from build123d import *
from OCP.BRepFilletAPI import BRepFilletAPI_MakeChamfer

# Parameters (mm, degrees)
ESBO_O1_W                = 16.6
ESBO_O1_H                = 16.6
RESSALTO_EXTRUS_O1_DEPTH = 40
ESBO_O2_W                = 50
ESBO_O2_H                = 65
RESSALTO_EXTRUS_O2_DEPTH = 50
ESBO_O3_W                = 30
ESBO_O3_H                = 40
CORTE_EXTRUS_O1_DEPTH    = 86.732140997
ESBO_O4_R                = 11.5
ESBO_O4_R_2              = 2.5
CORTE_EXTRUS_O2_DEPTH    = 78.821912081
ESBO_O5_W                = 18
ESBO_O5_H                = 5
CORTE_EXTRUS_O3_DEPTH    = 10
CHANFRO1_SIZE            = 25
CHANFRO1_SIZE2           = 16.23518983
FILETE2_R                = 10
ESBO_O8_W                = 18
ESBO_O8_H                = 5
CORTE_EXTRUS_O5_DEPTH    = 30
FILETE4_R                = 10
ESBO_O9_R                = 2.5
CORTE_EXTRUS_O7_DEPTH    = 70.207225056


with BuildPart() as part:
    # Esboço1 → Ressalto-extrusão1 (new body)
    with BuildSketch(Plane(origin=(0, 0, 0), x_dir=(1, 0, 0), z_dir=(0, 1, 0))):
        Rectangle(ESBO_O1_W, ESBO_O1_H)
    extrude(amount=RESSALTO_EXTRUS_O1_DEPTH)

    # Esboço2 → Ressalto-extrusão2 (add)
    with BuildSketch(Plane.XZ):
        Rectangle(ESBO_O2_W, ESBO_O2_H)
    extrude(amount=RESSALTO_EXTRUS_O2_DEPTH)

    # Esboço3 → Corte-extrusão1 (cut, through all)
    with BuildSketch(Plane.XY.offset(32.5)):
        with Locations((0, -30)):
            Rectangle(ESBO_O3_W, ESBO_O3_H)
    extrude(amount=-CORTE_EXTRUS_O1_DEPTH, mode=Mode.SUBTRACT)

    # Esboço4 → Corte-extrusão2 (cut, through all)
    with BuildSketch(Plane(origin=(25, 0, 0), x_dir=(0, 0, -1), z_dir=(1, 0, 0))):
        with Locations((0, -22)):
            Circle(ESBO_O4_R)
        with Locations((-23.8125, -22)):
            Circle(ESBO_O4_R_2)
        with Locations((23.8125, -22)):
            Circle(ESBO_O4_R_2)
        with Locations((-11.90625, -42.622229928)):
            Circle(ESBO_O4_R_2)
        with Locations((11.90625, -42.622229928)):
            Circle(ESBO_O4_R_2)
    extrude(amount=-CORTE_EXTRUS_O2_DEPTH, mode=Mode.SUBTRACT)

    # Esboço5 → Corte-extrusão3 (cut)
    with BuildSketch(Plane.ZY.offset(25)):
        with Locations((-23.5, -2.5)):
            Rectangle(ESBO_O5_W, ESBO_O5_H)
    extrude(amount=-CORTE_EXTRUS_O3_DEPTH, mode=Mode.SUBTRACT)

    # Chanfro1: one chamfer whose edges measure the first distance from different faces: ONE call of the kernel's chamfer builder (chamfer() names one face for all edges)
    chanfro1_edges_1 = [part.edges().sort_by_distance(p)[0] for p in [
        (20, -50, 32.5),
        (-20, -50, 32.5),
    ]]
    chanfro1_side_1 = [part.faces().sort_by_distance(p)[0] for p in [
        (0, -0.707106781, 32.5),
    ]]
    chanfro1_edges_2 = [part.edges().sort_by_distance(p)[0] for p in [
        (-20, -50, -32.5),
        (20, -50, -32.5),
    ]]
    chanfro1_side_2 = [part.faces().sort_by_distance(p)[0] for p in [
        (5, -0.707106781, -32.5),
    ]]
    chanfro1 = BRepFilletAPI_MakeChamfer(part.part.solid().wrapped)
    for e in chanfro1_edges_1:
        chanfro1.Add(CHANFRO1_SIZE, CHANFRO1_SIZE2, e.wrapped, chanfro1_side_1[0].wrapped)  # the first distance lies on this face
    for e in chanfro1_edges_2:
        chanfro1.Add(CHANFRO1_SIZE, CHANFRO1_SIZE2, e.wrapped, chanfro1_side_2[0].wrapped)  # the first distance lies on this face
    add(Compound.cast(chanfro1.Shape()), mode=Mode.REPLACE)

    # Filete2
    # the kernel refuses this fillet: 10 mm, written as the material it takes off along each edge
    with BuildSketch(Plane(origin=(7.594662626, -25, -32.5), x_dir=(0, 1, 0), z_dir=(1, 0, 0)), Plane(origin=(-32.405337374, -25, -32.5), x_dir=(0, 1, 0), z_dir=(1, 0, 0)), Plane(origin=(32.405337374, -25, 32.5), x_dir=(0, 1, 0), z_dir=(-1, 0, 0)), Plane(origin=(-7.594662626, -25, 32.5), x_dir=(0, 1, 0), z_dir=(-1, 0, 0))) as filete2_piece_1:
        with BuildLine():
            CenterArc((FILETE2_R * 0.296213494962, FILETE2_R), FILETE2_R, 237, 33)
            Line((-FILETE2_R * 0.248425540053, FILETE2_R * 0.161329432055), (0, 0))
            Line((0, 0), (FILETE2_R * 0.296213494962, 0))
        make_face()
    extrude(amount=24.810674748, mode=Mode.SUBTRACT)
    with BuildSketch(Plane(origin=(1.426107509, -50, -16.26481017), x_dir=(0, 0.8386705679454236, -0.5446390350150278), z_dir=(1, 0, 0)), Plane(origin=(-1.426107509, -50, 16.26481017), x_dir=(0, 0.8386705679454233, 0.5446390350150284), z_dir=(-1, 0, 0)), Plane(origin=(-38.573892491, -50, -16.26481017), x_dir=(0, 0.8386705679454236, -0.5446390350150278), z_dir=(1, 0, 0))) as filete2_piece_2:
        with BuildLine():
            CenterArc((FILETE2_R * 0.542955699638, FILETE2_R), FILETE2_R, 213, 57)
            Line((-FILETE2_R * 0.295714868307, FILETE2_R * 0.455360964985), (0, 0))
            Line((0, 0), (FILETE2_R * 0.542955699638, 0))
        make_face()
    extrude(amount=37.147784982, mode=Mode.SUBTRACT)
    with BuildSketch(Plane(origin=(38.573892491, -50, 16.26481017), x_dir=(0, 0, -1), z_dir=(-1, 0, 0))) as filete2_piece_3:
        with BuildLine():
            CenterArc((FILETE2_R * 0.542955699638, -FILETE2_R), FILETE2_R, 90, 57)
            Line((-FILETE2_R * 0.295714868307, -FILETE2_R * 0.455360964985), (0, 0))
            Line((0, 0), (FILETE2_R * 0.542955699638, 0))
        make_face()
    extrude(amount=37.147784982, mode=Mode.SUBTRACT)
    with BuildSketch(Plane(origin=(50, 0, 32.5), x_dir=(0, 0, -1), z_dir=(-1, 0, 0))) as filete2_piece_4:
        with BuildLine():
            CenterArc((FILETE2_R, FILETE2_R), FILETE2_R, 180, 90)
            Line((0, FILETE2_R), (0, 0))
            Line((0, 0), (FILETE2_R, 0))
        make_face()
    extrude(amount=100, mode=Mode.SUBTRACT)
    with BuildSketch(Plane(origin=(-50, -5, -32.5), x_dir=(0, -1, 0), z_dir=(1, 0, 0))) as filete2_piece_5:
        with BuildLine():
            CenterArc((FILETE2_R, -FILETE2_R), FILETE2_R, 90, 90)
            Line((0, -FILETE2_R), (0, 0))
            Line((0, 0), (FILETE2_R, 0))
        make_face()
    extrude(amount=35, mode=Mode.SUBTRACT)

    # Esboço8 → Corte-extrusão5 (cut)
    with BuildSketch(Plane.ZY.offset(15)):
        with Locations((-23.5, -2.5)):
            Rectangle(ESBO_O8_W, ESBO_O8_H)
        with Locations((-23.5, -7.5)):
            Rectangle(ESBO_O8_W, ESBO_O8_H)
    extrude(amount=-CORTE_EXTRUS_O5_DEPTH, mode=Mode.SUBTRACT)

    # Filete4
    filete4_edges = [part.edges().sort_by_distance(p)[0] for p in [
        (20, 0, -32.5),
    ]]
    fillet(filete4_edges, radius=FILETE4_R)

    # Esboço9 → Corte-extrusão7 (cut, through all)
    with BuildSketch(Plane(origin=(0, 0, 8.3), x_dir=(-1, 0, 0), z_dir=(0, 0, -1))):
        with Locations(Location((0, 10, 0), (0, 0, 180))):
            Circle(ESBO_O9_R)
        with Locations(Location((0, 35, 0), (0, 0, 180))):
            Circle(ESBO_O9_R)
    extrude(amount=CORTE_EXTRUS_O7_DEPTH, mode=Mode.SUBTRACT)


solid = part.part
Could you check a few things on this model? Use its own coordinates, in mm. A direction names the side the tool comes from. Give positions to 0.01 mm unless a question says otherwise; leave off trailing zeros. Write each loop counter-clockwise with the first axis right and the second up, starting at its lowest first coordinate (ties: lowest second). Pieces come first, ordered by that corner, then holes. Notation, with made-up numbers: (26, 50.25) -> (40, 50.25) arc R29 ccw to (40, 72.25) -> close; hole circle Ø3 at (51, 21.25). An arc over 180 degrees is marked (long way). Write each question's results on one line, items separated by ' | '. Start each with the question number.
Q1. Suppose I cut it at A-A, the plane y = 35. List the corners of the cut face in (x, z) for me, and give its area (3 significant figures).
Q2. Which directions (+Z, -Z, +X, -X, +Y, -Y) give clear straight access to the entire face, cutting with the end or side of a thin tool? Please do faces 5 (the face through (-20, -5, -19)), 6 (the face through (-19.93, -40.933, 13.749)).
Q3. I need wall thicknesses on probe 1 along Y at (x, z) = (0, 1); probe 2 along Y at (x, z) = (18, 0); probe 3 along X at (y, z) = (-31.5, 12). Which ranges of each line are inside material? Lowest first, please.
Q4. Suppose I cut it at B-B, the plane x = 0. List the corners of the cut face in (y, z) for me, and give its area (3 significant figures).
Q5. We'd pull the mould along Y, two halves only. Please class faces 1 (the face through (0, 40, 0)), 2 (the face through (20.07, -48.82, 15.55)), 3 (the face through (0, 20, -8.3)), 4 (the face through (-19.93, -40.933, -10.064)): +Y half, -Y half, draft (parallel to the pull), parting line (faces both ways), or undercut.
Q6. I'm going to push flat-ended pins straight in: pin 1 Ø8 at (x, y) = (1.5, -3) entering from -Z; pin 2 Ø13.5 at (y, z) = (18.5, 1.5) entering from +X; pin 3 Ø18.5 at (x, y) = (-1, 22.5) entering from +Z. Where does each tip first touch, or does it pass through?
Q7. Suppose I cut it at D-D, the plane x = -6. List the corners of the cut face in (y, z) for me, and give its area (3 significant figures).
Q8. Suppose I cut it at C-C, the plane z = -3. List the corners of the cut face in (x, y) for me, and give its area (3 significant figures).
Outcome:
1) outline: (-8.3, -8.3) -> (-2.5, -8.3) -> (-2.5, 8.3) -> (-8.3, 8.3) -> close; (2.5, -8.3) -> (8.3, -8.3) -> (8.3, 8.3) -> (2.5, 8.3) -> close | area: 193 mm2
2) face 5: -Z, -X, +Y | face 6: +X, -X
3) probe 1: -10 to 7.5, 12.5 to 32.5, 37.5 to 40 | probe 2: -50 to -33.5, -10.5 to 0 | probe 3: -25 to -15, 15 to 25
4) outline: (-10, -14.5) -> (0, -14.5) -> (0, -8.3) -> (7.5, -8.3) -> (7.5, 8.3) -> (0, 8.3) -> (0, 22.5) arc R10 ccw to (-10, 32.5) -> close; (12.5, -8.3) -> (32.5, -8.3) -> (32.5, 8.3) -> (12.5, 8.3) -> close; (37.5, -8.3) -> (40, -8.3) -> (40, 8.3) -> (37.5, 8.3) -> close | area: 947 mm2
5) face 1: +Y half | face 2: -Y half | face 3: draft | face 4: undercut
6) pin 1: z = -14.5 | pin 2: x = 8.3 | pin 3: z = 8.3
7) outline: (-10, -14.5) -> (0, -14.5) -> (0, -8.3) -> (40, -8.3) -> (40, 8.3) -> (0, 8.3) -> (0, 22.5) arc R10 ccw to (-10, 32.5) -> close | area: 1,110 mm2
8) outline: (-25, -50) -> (-15, -50) -> (-15, -33.1) -> (-25, -33.1) -> close; (-25, -10.9) -> (-15, -10.9) -> (-15, -10) -> (15, -10) -> (15, -10.9) -> (25, -10.9) -> (25, 0) -> (8.3, 0) -> (8.3, 40) -> (-8.3, 40) -> (-8.3, 0) -> (-25, 0) -> close; (15, -50) -> (25, -50) -> (25, -33.1) -> (15, -33.1) -> close; hole circle Ø5 at (0, 10); hole circle Ø5 at (0, 35) | area: 1,480 mm2
